Design review of the part built by this model. Coordinates are the model's own, in mm. Coordinates: 2 decimals unless noted, no trailing zeros. Loops run counter-clockwise (first coordinate to the right, second up) from the corner with the lowest first, then second, coordinate; pieces in that order, holes last.
Q1. Wall thickness on probe 1 along Y at (x, z) = (-0.4, 0.05); probe 2 along X at (y, z) = (0.5, 0.05): over which ranges is each line inside the solid? List them lowest first.
Q2. For P1, Ø0.7, axis at x = 0, z = 0, coming from the +Y side, flat-tipped, find the tip position at first contact; note if it passes through.
Q3. Add section B-B on y = 6. Give the boundary of the cut face in (x, z), and give its area (3 significant figures).
Q4. Add section A-A on x = 0. Give the boundary of the cut face in (y, z).
```python
from build123d import *

# Parameters (mm, degrees)
SKETCH1_R           = 1
BOSS_EXTRUDE1_DEPTH = 8
CHAMFER1_SIZE       = 0.25
CUT_EXTRUDE1_DEPTH  = 0.8


with BuildPart() as part:
    # Sketch1 → Boss-Extrude1 (new body)
    with BuildSketch(Plane(origin=(0, 0, 0), x_dir=(1, 0, 0), z_dir=(0, 1, 0))):
        Circle(SKETCH1_R)
    extrude(amount=BOSS_EXTRUDE1_DEPTH)

    # Chamfer1
    chamfer1_edges = [part.edges().sort_by_distance(p)[0] for p in [
        (-1, 0, 0),
    ]]
    chamfer(chamfer1_edges, length=CHAMFER1_SIZE)

    # Sketch2 → Cut-Extrude1 (cut)
    with BuildSketch(Plane(origin=(0, 8, 0), x_dir=(1, 0, 0), z_dir=(0, 1, 0))):
        Polygon((0.259807621, -0.45), (0.519615242, 0), (0.259807621, 0.45), (-0.259807621, 0.45), (-0.519615242, 0), (-0.259807621, -0.45), align=None)
    extrude(amount=-CUT_EXTRUDE1_DEPTH, mode=Mode.SUBTRACT)


solid = part.part
```
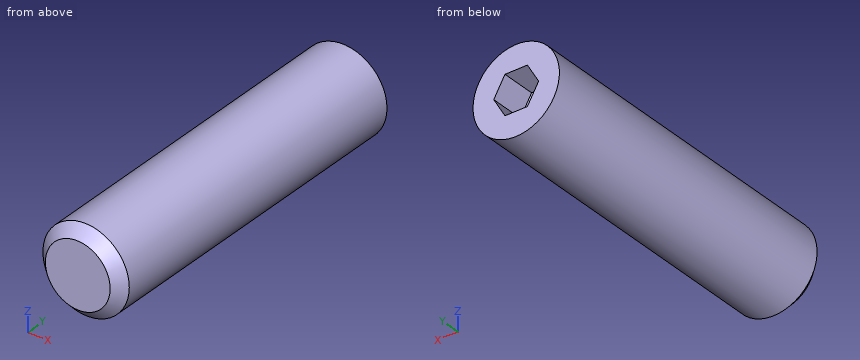
Entries:
1. probe 1: y = 0 to 7.2
1. probe 2: x = -1 to 1
2. P1: stops at y = 7.2
3. outline: circle Ø2 at (0, 0)
3. area: 3.14 mm2
4. outline: (0, -0.75) - (0.25, -1) - (8, -1) - (8, -0.45) - (7.2, -0.45) - (7.2, 0.45) - (8, 0.45) - (8, 1) - (0.25, 1) - (0, 0.75) - close
